from build123d import *

# Parameters (mm, degrees)
EXTRUDE_1_DEPTH     = 30
EXTRUDE_2_DEPTH     = 10
CUT_EXTRUDE_1_DEPTH = 70


with BuildPart() as part:
    # 草圖1 → 填料-伸長1 (new body)
    with BuildSketch(Plane.XY):
        Polygon((-40, 0), (40, 0), (30, 10), (20, 10), (20, 40), (-20, 40), (-20, 10), (-30, 10), align=None)
    extrude(amount=EXTRUDE_1_DEPTH)

    # 草圖2 → 填料-伸長2 (add)
    with BuildSketch(Plane.XY.offset(30)):
        with BuildLine():
            Line((-20, 40), (20, 40))
            ThreePointArc((20, 40), (0, 19.871866441), (-20, 40))
        make_face()
    extrude(amount=EXTRUDE_2_DEPTH)

    # 草圖3 → 除料-伸長1 (cut)
    with BuildSketch(Plane.XY.offset(40)):
        with BuildLine():
            Line((10, 40), (-10, 40))
            ThreePointArc((-10, 40), (0, 30), (10, 40))
        make_face()
    extrude(amount=-CUT_EXTRUDE_1_DEPTH, mode=Mode.SUBTRACT)


solid = part.part
Could you check a few things on this model? Use its own coordinates, in mm. A direction names the side the tool comes from. Coordinates: 2 decimals unless noted, no trailing zeros. Order: outer loops, then holes, each group sorted by start corner. A loop starts at its lowest first (then second) coordinate and runs counter-clockwise, first axis right, second up.
Q1. Will these pins go through, and if not, where does the flat tip stop? pin 1 (2 mm diameter, centred on y = 30.5, z = 34.5, fed in from -X); pin 2 (12 mm diameter, centred on x = 25.5, y = 18.5, fed in from -Z); pin 3 (9 mm diameter, centred on y = 26, z = 21, fed in from -X); pin 4 (3 mm diameter, centred on y = 31, z = 6.5, fed in from +X).
Q2. Suppose I cut it at C-C on y = 15. Please give me the cut outline in (x, z).
Q3. Please list where these lines run through material, in increasing order: L1, parallel to Z at x = 10.5, y = 9; L2, parallel to X at y = 26, z = 12.
Q4. Suppose I cut it at A-A on z = 23. Please give me the cut outline in (x, y), and give its area (3 significant figures).
Q5. Which directions (+Z, -Z, +X, -X, +Y, -Y) give clear straight access to the entire face, cutting with the end or side of a thin tool? Please do faces 1 (the flat face through (25, 10, 15)), 2 (the flat face through (-25, 10, 15)), 3 (the cylindrical face through (0, 30, 20)).
Q6. Suppose I cut it at D-D on y = 21. Please give me the cut outline in (x, z), and give its area (3 significant figures).
Q7. Suppose I cut it at B-B on x = 0. Please give me the cut outline in (y, z), and give its area (3 significant figures).
Answer:
1. pin 1: stops at x = -18.16
1. pin 2: stops at z = 0
1. pin 3: stops at x = -20
1. pin 4: stops at x = 20
2. outline: (-20, 0) - (20, 0) - (20, 30) - (-20, 30) - close
3. L1: z = 0 to 30
3. L2: x = -20 to 20
4. outline: (-40, 0) - (40, 0) - (30, 10) - (20, 10) - (20, 40) - (10, 40) arc R10 cw to (-10, 40) - (-20, 40) - (-20, 10) - (-30, 10) - close
4. area: 1,740 mm2
5. face 1: +Z, -Z, +X, +Y
5. face 2: +Z, -Z, -X, +Y
5. face 3: +Z, -Z, +Y
6. outline: (-20, 0) - (20, 0) - (20, 30) - (6.62, 30) - (6.62, 40) - (-6.62, 40) - (-6.62, 30) - (-20, 30) - close
6. area: 1,330 mm2
7. outline: (0, 0) - (30, 0) - (30, 40) - (19.87, 40) - (19.87, 30) - (0, 30) - close
7. area: 1,000 mm2
